Work out the finished part from the listing and answer in its coordinate system (mm). A direction names the side the tool comes from. Give positions to 0.01 mm unless a question says otherwise; leave off trailing zeros. Write each loop counter-clockwise with the first axis right and the second up, starting at its lowest first coordinate (ties: lowest second). Pieces come first, ordered by that corner, then holes. Notation, with made-up numbers: (76, 73) -> (124, 73) arc R31 cw to (124, 106) -> close; hole circle Ø11 at (59, 79). An arc over 180 degrees is marked (long way). Use a Markdown table: item, result. Add a question column.
Q1. For a pull along Z with two mould halves and no side action, classify faces 5 (the face through (0, -10, 21.165)), 6 (the face through (-1.5, -25.2, 1.2)), 7 (the face through (0.021, -3.902, 18.309)) as pulls with the +Z half, pulls with the -Z half, needs draft (parallel to the pull), parting line crosses it, or undercut.
Q2. Consider line 1 (Y direction, x = 0.7, z = -10); line 2 (Y direction, x = 1.3, z = -5); line 3 (Z direction, x = 0.5, y = -12). Determine where each line is inside the solid, lowest interval first.
Q3. Section A-A, the plane x = 0.8 is taken. Give the vertices of the cut face in (y, z).
Q4. Section C-C, the plane y = -10.5 is taken. Give the vertices of the cut face in (x, z).
Q5. Each of these flat-tipped pins is pushed along its axis until it touches: pin 1 Ø1 at (x, z) = (0, 3) entering from -Y; pin 2 Ø0.9 at (x, z) = (0.5, 11) entering from -Y; pin 3 Ø1.6 at (x, z) = (0.5, 20) entering from -Y. Where does it stop, or does it pass through?
Q6. Section B-B, the plane z = 1 is taken. Give the vertices of the cut face in (x, y).
Q7. For faces 1 (the face through (0, -11, 19.165)), 2 (the face through (-0.021, -1.504, 19.739)), 3 (the face through (0.02, -3.94, 4.03)), 4 (the face through (0, -52.97, 3)), determine the directions among +Z, -Z, +X, -X, +Y, -Y from which every point of the face is accessible in a straight line to the end or side of a thin tool.
Q8. Section D-D, the plane z = 12.5 is taken. Give the vertices of the cut face in (x, y).
from build123d import *

# Parameters (mm, degrees)
F1_DEPTH = 1.5
F2_R     = 3
F3_R     = 1
F4_R     = 5


with BuildPart() as f1:
    # F0 (on Right) → F1 (new body, symmetric)
    with BuildSketch(Plane.YZ):
        Polygon((-15, 19.164762), (-3, 19.164762), (-3, 3.104762), (-52.969541, 4.849737), (-52.969541, 1.849737), (-46.973196, 1.64034), (-5.996345, 0.209397), (0, 0), (0, 21.164762), (-15, 21.164762), align=None)
        Polygon((-1.256382, -35.97807), (0, 0), (-5.996345, 0.209397), (-7.252727, -35.768673), align=None)
        Polygon((-46.973196, 1.64034), (-52.969541, 1.849737), (-54.225923, -34.128333), (-48.229578, -34.33773), align=None)
    extrude(amount=F1_DEPTH, both=True)

    # F2
    f2_edges = [f1.edges().sort_by_distance(p)[0] for p in [
        (0, -3, 19.164762),
        (0, -3, 3.104762),
    ]]
    fillet(f2_edges, radius=F2_R)

    # F3
    f3_edges = [f1.edges().sort_by_distance(p)[0] for p in [
        (0, -52.969541, 4.849737),
    ]]
    fillet(f3_edges, radius=F3_R)

    # F4
    f4_edges = [f1.edges().sort_by_distance(p)[0] for p in [
        (0, 0, 21.164762),
    ]]
    fillet(f4_edges, radius=F4_R)


solid = f1.part
Result set:
| question | item | result |
|---|---|---|
| 1 | face 5 | pulls with the +Z half |
| 1 | face 6 | needs draft |
| 1 | face 7 | undercut |
| 2 | line 1 | y = -53.38 to -47.38, -6.35 to -0.35 |
| 2 | line 2 | y = -53.21 to -47.21, -6.18 to -0.17 |
| 2 | line 3 | z = 0.42 to 3.42, 19.16 to 21.16 |
| 3 | outline | (-54.23, -34.13) -> (-48.23, -34.34) -> (-46.97, 1.64) -> (-6, 0.21) -> (-7.25, -35.77) -> (-1.26, -35.98) -> (0, 0) -> (0, 16.16) arc R5 ccw to (-5, 21.16) -> (-15, 21.16) -> (-15, 19.16) -> (-6, 19.16) arc R3 cw to (-3, 16.16) -> (-3, 6.21) arc R3 cw to (-6.1, 3.21) -> (-51.93, 4.81) arc R1 ccw to (-52.97, 3.81) -> (-52.97, 1.85) -> close |
| 4 | outline | (-1.5, 0.37) -> (1.5, 0.37) -> (1.5, 3.37) -> (-1.5, 3.37) -> close; (-1.5, 19.16) -> (1.5, 19.16) -> (1.5, 21.16) -> (-1.5, 21.16) -> close |
| 5 | pin 1 | stops at y = -52.97 |
| 5 | pin 2 | stops at y = -3 |
| 5 | pin 3 | stops at y = -15 |
| 6 | outline | (-1.5, -53) -> (1.5, -53) -> (1.5, -47) -> (-1.5, -47) -> close; (-1.5, -28.64) -> (1.5, -28.64) -> (1.5, 0) -> (-1.5, 0) -> close |
| 7 | face 1 | +X, -X, -Y |
| 7 | face 2 | +Z, +X, -X, +Y |
| 7 | face 3 | +X, -X |
| 7 | face 4 | +Z, +X, -X, -Y |
| 8 | outline | (-1.5, -3) -> (1.5, -3) -> (1.5, 0) -> (-1.5, 0) -> close |
